from build123d import *

# Parameters (mm, degrees)
SKETCH_1_W = 15
SKETCH_1_H = 2
FILLET_1_R = 10


with BuildPart() as part:
    # 草图1 → 旋转1 (revolve)
    with BuildSketch(Plane(origin=(0, 0, 0), x_dir=(1, 0, 0), z_dir=(0, 1, 0))):
        Polygon((-22.158783784, -3.392857143), (-20.158783784, -3.392857143), (-20.158783784, 1.857142857), (-20.158783784, 2.857142857), (-22.158783784, 2.857142857), align=None)
        Polygon((-20.158783784, -3.392857143), (-5.658783784, -3.392857143), (-5.658783784, -1.392857143), (-5.658783784, 1.857142857), (-20.158783784, 1.857142857), align=None)
        with Locations((1.841216216, -2.392857143)):
            Rectangle(SKETCH_1_W, SKETCH_1_H)
    revolve(axis=Axis((9.341216216, 0, 3.392857143), (-1, 0, 0)))

    # 圆角1
    # the kernel refuses this fillet: 10 mm, written as the material it adds along each edge
    with BuildSketch(Plane(origin=(-5.658783784, 0, 3.392857143), x_dir=(0, 0, -1), z_dir=(0, 1, 0))) as fillet_1_piece_1:
        with BuildLine():
            CenterArc((12, -7.378177282), FILLET_1_R, 132.454150204, 47.545849796)
            Line((2, -7.378177282), (1.8, -7.378177282))
            Line((1.8, -7.378177282), (1.8, 0))
            Line((1.8, 0), (2, 0.2))
            ThreePointArc((2, 0.2), (3.625, 0.2), (5.115, 0.147563546))
            Line((5.115, 0.147563546), (5.25, 0))
        make_face()
    revolve(axis=Axis((-5.658783784, 0, 3.392857143), (-1, 0, 0)))


solid = part.part
Check sheet for the modelled part. Datum: model origin and axes. Units: mm. A direction names the side the tool comes from. Round coordinates to 2 decimals unless told otherwise and drop trailing zeros. Loops run counter-clockwise (first coordinate to the right, second up) from the corner with the lowest first, then second, coordinate; pieces in that order, holes last. Notation, with made-up numbers: (78.25, -23) - (110.25, -23) arc R36 ccw to (110.25, 14) - close; hole circle Ø6 at (50, -29). An arc over 180 degrees is marked (long way). Answer as CSV lines item,"result". Start each with the question number.
Item 1: Section check B-B (x = -16). Record the boundary of the cut face in (y, z).
Item 2: Section check D-D (y = 5.75). Record the boundary of the cut face in (x, z), and give its area (3 significant figures).
Item 3: Scan lines: line 1 (X direction, y = 5.75, z = 4.5); line 2 (Z direction, x = -5.5, y = 3.75); line 3 (Y direction, x = -7.5, z = 4). Record each from-to range of solid material in increasing order. Write a range as [from, to].
Item 4: Set-up check for faces 1 (the flat face through (9.341, 0, 3)), 2 (the flat face through (-20.159, 1, -2)): record each of +Z, -Z, +X, -X, +Y, -Y from which the full face is reachable in a straight line by a thin tool's end or side.
Item 5: Section check A-A (y = 0). Record the boundary of the cut face in (x, z).
Item 6: Section check C-C (x = 1). Record the boundary of the cut face in (y, z).
Item 7: Depth check by flat-ended pin: P1, Ø1.5, axis at x = -9.5, y = 4.5, coming from the +Z side; P2, Ø1, axis at x = -18, y = 4.5, coming from the +Z side. Enter the tip coordinate at first touch or a pass-through.
Report:
1,outline,"circle Ø10.5 at (0, 3.39)"
2,outline,"(-22.16, 0.94) - (-20.16, 0.94) - (-20.16, 5.84) - (-22.16, 5.84) - close"
2,area,"9.80 mm2"
3,line 1,"x = [-22.16, -20.16]"
3,line 2,"z = [-0.03, 6.82]"
3,line 3,"y = [-5.21, 5.21]"
4,face 1,"+Z, -Z, +X, +Y, -Y"
4,face 2,"+X"
5,outline,"(-22.16, -2.86) - (-20.16, -2.86) - (-20.16, -1.86) - (-5.66, -1.86) arc R10 cw to (1.72, 1.39) - (9.34, 1.39) - (9.34, 5.39) - (1.72, 5.39) arc R10 cw to (-5.66, 8.64) - (-20.16, 8.64) - (-20.16, 9.64) - (-22.16, 9.64) - close"
6,outline,"circle Ø4.05 at (0, 3.39)"
7,P1,"stops at z = 7.07"
7,P2,"stops at z = 6.79"
